Here's how the part is built. I have some questions about the finished solid (model axes, mm). A direction names the side the tool comes from. Coordinates: 2 decimals unless noted, no trailing zeros. Write each loop counter-clockwise with the first axis right and the second up, starting at its lowest first coordinate (ties: lowest second). Pieces come first, ordered by that corner, then holes. Notation, with made-up numbers: (10, -39) -> (48, -39) arc R21 ccw to (48, -7) -> close; hole circle Ø3 at (37.25, 30). An arc over 180 degrees is marked (long way). Use a Markdown table: item, result. Add a question column.
Item 1: Imagine slicing it at B-B, the plane y = -7.5. Write out the boundary of the cut face in (x, z).
Item 2: Will these pins go through, and if not, where does the flat tip stop? pin 1 Ø2.5 at (y, z) = (-12.5, 10) entering from -X; pin 2 Ø2 at (x, y) = (-11, -7) entering from +Z; pin 3 Ø5.5 at (y, z) = (-12, 10) entering from +X.
Item 3: If I drill on line 1 along Y through (x, z) = (12, 4.25); line 2 along X through (y, z) = (-11.5, 8.5); line 3 along X through (y, z) = (-17.5, 4.75), over which ranges is the centre line in solid material (lowest first)? Write a range as from..to.
Item 4: If we mould it in two halves opening along X, with no side actions, what happens to faces 6 (the flat face through (-11, -11, 0)), 7 (the cylindrical face through (8.918, -22.498, 9.073)), 8 (the cylindrical face through (13.53, -4.62, 3.37))? For each: pulls with the +X half, pulls with the -X half, needs draft (parallel to the pull), parting line crosses it, or undercut.
Item 5: Imagine slicing it at A-A, the plane z = 4.25. Write out the boundary of the cut face in (x, y) (3 decimals), and give its area (3 significant figures).
Item 6: Imagine slicing it at D-D, the plane x = -1. Write out the boundary of the cut face in (y, z).
Item 7: Imagine slicing it at C-C, the plane z = 10.25. Write out the boundary of the cut face in (x, y), and give its area (3 significant figures).
Item 8: On a 3-axis mill with a long thin cutter (end or side, diameter ignored), from which of +Z, -Z, +X, -X, +Y, -Y can I reach the whole of each face in a straight line? I mean faces 1 (the cylindrical face through (-8.918, -22.498, 9.007)), 2 (the cylindrical face through (8.938, -0.382, 9.073)), 3 (the flat face through (9.3, -11, 9)), 4 (the cylindrical face through (-8.938, -0.382, 9.007)), 5 (the flat face through (0, -11, 9.52)). Say none if no direction works.
```python
from build123d import *

# Parameters (mm, degrees)
F1_DEPTH = 22.86
F2_R     = 1.27
F3_R     = 1.524
F4_DEPTH = 6.65
F5_R     = 1.27


with BuildPart() as f1:
    # F0 (on Front) → F1 (new body)
    with BuildSketch(Plane.XZ):
        Polygon((-14.85, 6.65), (-14.85, 0), (-6.5, 0), (-6.5, 9.52), (0, 9.52), (0, 12.7), (-9.3, 12.7), (-9.3, 6.65), align=None)
        Polygon((0, 12.7), (0, 9.52), (6.5, 9.52), (6.5, 0), (14.85, 0), (14.85, 6.65), (9.3, 6.65), (9.3, 12.7), align=None)
    extrude(amount=F1_DEPTH)

    # F2
    f2_edges = [f1.edges().sort_by_distance(p)[0] for p in [
        (9.3, -11.43, 12.7),
        (-9.3, -11.43, 12.7),
    ]]
    fillet(f2_edges, radius=F2_R)

    # F3 (on face) → F4 (cut, through all)
    with BuildSketch(Plane.XY.offset(6.65)):
        with BuildLine():
            ThreePointArc((-10.551, -5.08), (-10.997369, -4.002369), (-12.075, -3.556))
            Line((-12.075, -3.556), (-12.075, -5.08))
            Line((-12.075, -5.08), (-12.075, -6.604))
            ThreePointArc((-12.075, -6.604), (-10.997369, -6.157631), (-10.551, -5.08))
        make_face()
        with BuildLine():
            ThreePointArc((-10.551, -17.78), (-10.997369, -16.702369), (-12.075, -16.256))
            Line((-12.075, -16.256), (-12.075, -17.78))
            Line((-12.075, -17.78), (-12.075, -19.304))
            ThreePointArc((-12.075, -19.304), (-10.997369, -18.857631), (-10.551, -17.78))
        make_face()
        with BuildLine():
            Line((-12.075, -17.78), (-12.075, -16.256))
            ThreePointArc((-12.075, -16.256), (-13.599, -17.78), (-12.075, -19.304))
            Line((-12.075, -19.304), (-12.075, -17.78))
        make_face()
        with BuildLine():
            Line((-12.075, -5.08), (-12.075, -3.556))
            ThreePointArc((-12.075, -3.556), (-13.599, -5.08), (-12.075, -6.604))
            Line((-12.075, -6.604), (-12.075, -5.08))
        make_face()
        with Locations((12.075, -5.08)):
            Circle(F3_R)
        with Locations((12.075, -17.78)):
            Circle(F3_R)
    extrude(amount=-F4_DEPTH, mode=Mode.SUBTRACT)

    # F5
    f5_edges = [f1.edges().sort_by_distance(p)[0] for p in [
        (14.85, 0, 3.325),
        (9.3, 0, 9.04),
        (-14.85, 0, 3.325),
        (-9.3, -22.86, 9.04),
        (-14.85, -22.86, 3.325),
        (14.85, -22.86, 3.325),
    ]]
    fillet(f5_edges, radius=F5_R)


solid = f1.part
```
Ans:
| question | item | result |
|---|---|---|
| 1 | outline | (-14.85, 0) -> (-6.5, 0) -> (-6.5, 9.52) -> (6.5, 9.52) -> (6.5, 0) -> (14.85, 0) -> (14.85, 6.65) -> (9.3, 6.65) -> (9.3, 11.43) arc R1.27 ccw to (8.03, 12.7) -> (-8.03, 12.7) arc R1.27 ccw to (-9.3, 11.43) -> (-9.3, 6.65) -> (-14.85, 6.65) -> close |
| 2 | pin 1 | stops at x = -9.3 |
| 2 | pin 2 | stops at z = 6.65 |
| 2 | pin 3 | stops at x = 9.3 |
| 3 | line 1 | y = -22.86..-19.3, -16.26..-6.6, -3.56..0 |
| 3 | line 2 | x = -9.3..-6.5, 6.5..9.3 |
| 3 | line 3 | x = -14.85..-13.57, -10.58..-6.5, 6.5..10.58, 13.57..14.85 |
| 4 | face 6 | needs draft |
| 4 | face 7 | pulls with the +X half |
| 4 | face 8 | undercut |
| 5 | outline | (-14.85, -21.59) arc R1.27 ccw to (-13.58, -22.86) -> (-6.5, -22.86) -> (-6.5, 0) -> (-13.58, 0) arc R1.27 ccw to (-14.85, -1.27) -> close; (6.5, -22.86) -> (13.58, -22.86) arc R1.27 ccw to (14.85, -21.59) -> (14.85, -1.27) arc R1.27 ccw to (13.58, 0) -> (6.5, 0) -> close; hole (-12.075, -16.256) arc R1.524 ccw (long way) to (-10.551, -17.78) arc R1.524 ccw to start; hole (-12.075, -3.556) arc R1.524 ccw (long way) to (-10.551, -5.08) arc R1.524 ccw to start; hole circle Ø3.048 at (12.075, -17.78); hole circle Ø3.048 at (12.075, -5.08) |
| 5 | area | 351 mm^2 |
| 6 | outline | (-22.86, 9.52) -> (0, 9.52) -> (0, 11.43) arc R1.27 ccw to (-1.27, 12.7) -> (-21.59, 12.7) arc R1.27 ccw to (-22.86, 11.43) -> close |
| 7 | outline | (-9.3, -21.59) arc R1.27 ccw to (-8.03, -22.86) -> (8.03, -22.86) arc R1.27 ccw to (9.3, -21.59) -> (9.3, -1.27) arc R1.27 ccw to (8.03, 0) -> (-8.03, 0) arc R1.27 ccw to (-9.3, -1.27) -> close |
| 7 | area | 424 mm^2 |
| 8 | face 1 | +Z, -X, -Y |
| 8 | face 2 | +Z, +X, +Y |
| 8 | face 3 | +Z, +X, +Y, -Y |
| 8 | face 4 | +Z, -X, +Y |
| 8 | face 5 | -Z, +Y, -Y |
